Read the model definition and answer for the solid it produces. Units are mm, in the model's axes. A direction names the side the tool comes from. Coordinates: 2 decimals unless noted, no trailing zeros. Loops run counter-clockwise (first coordinate to the right, second up) from the corner with the lowest first, then second, coordinate; pieces in that order, holes last. Notation, with made-up numbers: M -27,69.25 L -16,69.25 A28 ccw -16,97.25 Z; hole C 11.25,15.5 d6. An arc over 180 degrees is marked long. One line per item, written item: value. Start each with the question number.
1. The part is cut by section A-A (x = 113). Write down the section's boundary in (y, z), then the cut area to 3 significant figures.
2. For faces 4 (the face through (120, -11.5, 2)), 5 (the face through (75, 14, 2)), 6 (the face through (-120, -5, 2)), determine the directions among +Z, -Z, +X, -X, +Y, -Y from which every point of the face is accessible in a straight line to the end or side of a thin tool.
3. The part is cut by section B-B (x = -78.5). Write down the section's boundary in (y, z).
4. Consider probe 1 along Y at (x, z) = (113, 2.4); probe 2 along X at (y, z) = (13.5, 2.85); probe 3 along X at (y, z) = (-2, 2). Determine where each line is inside the solid, lowest interval first.
5. Flat-ended cylindrical pins translate along their axes: pin 1 (1.8 mm diameter, centred on x = -127, z = 1.5, fed in from +Y); pin 2 (1 mm diameter, centred on y = 2, z = 2.5, fed in from +X); pin 3 (1.2 mm diameter, centred on x = 92.5, z = 1.5, fed in from -Y); pin 4 (1.5 mm diameter, centred on x = 51, y = 2.5, fed in from +Z). Find the tip coordinate at first contact, or state that the pin passes through.
6. The part is cut by section C-C (z = 3). State how many separate pieces and enclosed holes the cut face has, then the cut area to 3 significant figures.
7. Determine the mould class of faces 1 (the face through (110, -9, 2)), 2 (the face through (-83, -2.5, 2)), 3 (the face through (126, -4, 2)) for opening direction X: +X half, -X half, draft (parallel to the pull), parting line (faces both ways), or undercut.
Autodesk Inventor part; units mm, degrees
ref_plane "YZ Plane" through (0, 0, 0) normal (1, 0, 0) x (0, 1, 0)
ref_plane "XZ Plane" through (0, 0, 0) normal (0, 1, 0) x (-1, 0, 0)
ref_plane "XY Plane" through (0, 0, 0) normal (0, 0, 1) x (1, 0, 0)
sketch "Sketch1" plane through (0, 0, 0) normal (0, 0, 1) x (1, 0, 0)
  line L0 (-130, 16.5) -> (130, 16.5)
  line L1 (130, 16.5) -> (130, -16.5)
  line L2 (130, -16.5) -> (-130, -16.5)
  line L3 (-130, -16.5) -> (-130, 16.5)
  point P0 (0, 0)
  dimension "d0" = 260
  dimension "d1" = 33
  dimension "d2" = 16.5
  dimension "d3" = 130
extrude "Base" add sketch "Sketch1" along normal blind 4
sketch "Sketch2" plane through (0, 0, 4) normal (0, 0, 1) x (1, 0, 0)
  line L0 (130, 16.5) -> (130, -16.5)
  line L1 (-130, 16.5) -> (130, 16.5)
  line L2 (-130, -16.5) -> (-130, 16.5)
  line L3 (130, -16.5) -> (-130, -16.5)
  line L4 (75, 16.5) -> (110, 16.5)
  line L5 (110, 16.5) -> (110, 12.5)
  line L6 (110, 12.5) -> (75, 12.5)
  line L7 (75, 12.5) -> (75, 16.5)
  line L8 (-130, 16.5) -> (55, 16.5)
  line L9 (55, 16.5) -> (55, 12.5)
  line L10 (55, 12.5) -> (-130, 12.5)
  line L11 (-130, 12.5) -> (-130, 16.5)
  line L12 (35, -7.5) -> (55, -7.5)
  line L13 (55, -7.5) -> (55, -16.5)
  line L14 (55, -16.5) -> (35, -16.5)
  line L15 (35, -16.5) -> (35, -7.5)
  line L16 (75, -7.5) -> (110, -7.5)
  line L17 (110, -7.5) -> (110, -16.5)
  line L18 (110, -16.5) -> (75, -16.5)
  line L19 (75, -16.5) -> (75, -7.5)
  line L20 (110, -11.5) -> (130, -11.5)
  line L21 (130, -11.5) -> (130, -16.5)
  line L22 (130, -16.5) -> (110, -16.5)
  line L23 (110, -16.5) -> (110, -11.5)
  line L24 (55, -11.5) -> (75, -11.5)
  line L25 (75, -11.5) -> (75, -16.5)
  line L26 (75, -16.5) -> (55, -16.5)
  line L27 (55, -16.5) -> (55, -11.5)
  point P0 (0, 0)
  dimension "d6" = 35
  dimension "d7" = 4
  dimension "d8" = 0
  dimension "d9" = 20
  dimension "d10" = 185
  dimension "d11" = 4
  dimension "d12" = 0
  dimension "d13" = 0
  dimension "d14" = 20
  dimension "d15" = 20
  dimension "d16" = 9
  dimension "d17" = 0
  dimension "d18" = 165
  dimension "d19" = 35
  dimension "d20" = 9
  dimension "d21" = 0
  dimension "d22" = 20
  dimension "d23" = 20
  dimension "d24" = 5
  dimension "d25" = 20
  dimension "d26" = 5
  dimension "d27" = 0
  dimension "d28" = 0
  dimension "d29" = 0
  dimension "d30" = 0
  dimension "d98" = 20
extrude "StructureMounting" cut sketch "Sketch2" against normal blind 4 contours L0 L3 L17 L20 | L5 L6 L7 L1 | L17 L3 L19 L16 | L9 L10 L2 L1 | L3 L13 L24 L19 | L3 L15 L12 L13
sketch "Sketch4" plane through (0, 0, 4) normal (0, 0, 1) x (1, 0, 0)
  line L0 (55, 12.5) -> (-130, 12.5)
  line L1 (-130, -16.5) -> (-130, 12.5)
  line L2 (35, -16.5) -> (-130, -16.5)
  line L3 (35, -16.5) -> (35, -7.5)
  line L4 (55, 16.5) -> (55, 12.5)
  line L5 (35, -7.5) -> (-130, -16.5)
  line L6 (-130, 3.5) -> (35, 12.5)
  point P0 (0, 0)
  dimension "d42" = 20
  dimension "d43" = 20
extrude "MotorRamp" cut sketch "Sketch4" against normal blind 4
sketch "Sketch5" plane through (0, 0, 4) normal (0, 0, 1) x (1, 0, 0)
  line L0 (110, 12.5) -> (75, 12.5)
  line L1 (75, 12.5) -> (75, 16.5)
  line L2 (94.274, 12.5) -> (98.274, 12.5)
  line L3 (98.274, 12.5) -> (98.274, 2.5)
  line L4 (98.274, 2.5) -> (94.274, 2.5)
  line L5 (94.274, 2.5) -> (94.274, 12.5)
  line L6 (110, 16.5) -> (110, 12.5)
  point P0 (0, 0)
  dimension "d46" = 4
  dimension "d47" = 10
  dimension "d48" = 0
  dimension "d49" = 19.274
  dimension "d100" = 11.726
extrude "LowSleeve" [suppressed]
sketch "Sketch6" plane through (0, 0, 4) normal (0, 0, 1) x (1, 0, 0)
  line L0 (-130, -16.5) -> (-130, 3.5)
  line L1 (-120, -2.5) -> (-105, -2.5)
  line L2 (-105, -2.5) -> (-105, -6.5)
  line L3 (-105, -6.5) -> (-120, -6.5)
  line L4 (-120, -6.5) -> (-120, -2.5)
  line L5 (-90, -2.5) -> (-75, -2.5)
  line L6 (-75, -2.5) -> (-75, -6.5)
  line L7 (-75, -6.5) -> (-90, -6.5)
  line L8 (-90, -6.5) -> (-90, -2.5)
  line L9 (98.274, 2.5) -> (94.274, 2.5)
  line L10 (-106.4171, -4.5) -> (-87.4505, -4.5) construction
  circle A0 centre (-97.5, -4.5) radius 1.25
  point P0 (0, 0)
  dimension "d63" = 15
  dimension "d64" = 4
  dimension "d67" = 30
  dimension "d72" = 10
  dimension "d73" = 10
  dimension "d166" = 2
  dimension "d167" = 2.5
  dimension "d168" = 7.5
extrude "MotorSleeves" cut sketch "Sketch6" against normal blind 4
sketch "Sketch10" plane through (0, 0, 4) normal (0, 0, 1) x (1, 0, 0)
  line L0 (130, 16.5) -> (130, -11.5)
  line L1 (122, 6) -> (130, 6)
  line L2 (130, 6) -> (130, -4)
  line L3 (130, -4) -> (122, -4)
  line L4 (122, -4) -> (122, 6)
  point P0 (0, 0)
  dimension "d109" = 8
  dimension "d110" = 10
  dimension "d111" = 0
  dimension "d112" = 4
extrude "Cabling" cut sketch "Sketch10" against normal blind 4
sketch "Sketch12" plane through (0, 0, 4) normal (0, 0, 1) x (1, 0, 0)
  line L0 (35, 12.5) -> (-130, 3.5)
  line L1 (-0.084, 8.5834) -> (19.8863, 9.6726)
  line L2 (19.8863, 9.6726) -> (20.1041, 5.6786)
  line L3 (20.1041, 5.6786) -> (0.1338, 4.5893)
  line L4 (0.1338, 4.5893) -> (-0.084, 8.5834)
  point P0 (0, 0)
  dimension "d124" = 4
  dimension "d125" = 20
  dimension "d126" = 2
  dimension "d127" = 130
extrude "ESCholder" cut sketch "Sketch12" against normal blind 4
sketch "Sketch13" plane through (0, 0, 4) normal (0, 0, 1) x (1, 0, 0)
  line L0 (55, 16.5) -> (55, 12.5)
  line L1 (55, 12.5) -> (35, 12.5)
  line L2 (35, 12.5) -> (-130, 3.5)
  line L3 (-130, -16.5) -> (35, -7.5)
  line L4 (-30.0123, 6.4502) -> (-26.0182, 6.668)
  line L5 (-26.0182, 6.668) -> (-25.7459, 1.6754)
  line L6 (-25.7459, 1.6754) -> (-29.7399, 1.4576)
  line L7 (-29.7399, 1.4576) -> (-30.0123, 6.4502)
  line L8 (-47.5366, -2.0169) -> (-6.9954, 0.1945) construction
  line L9 (-29.1953, -8.5276) -> (-25.2012, -8.3097)
  line L10 (-25.2012, -8.3097) -> (-25.4736, -3.3171)
  line L11 (-25.4736, -3.3171) -> (-29.4676, -3.535)
  line L12 (-29.4676, -3.535) -> (-29.1953, -8.5276)
  line L13 (20.1041, 5.6786) -> (0.1338, 4.5893)
  line L14 (-27.9377, 5.1382) -> (-27.2725, -7.0585) construction
  circle A0 centre (-27.6051, -0.9601) radius 1.25
  line L15 (49, 10) -> (53, 10)
  line L16 (53, 10) -> (53, 5)
  line L17 (53, 5) -> (49, 5)
  line L18 (49, 5) -> (49, 10)
  line L19 (39.5253, 2.5) -> (63.8345, 2.5) construction
  line L20 (49, -5) -> (53, -5)
  line L21 (53, -5) -> (53, 0)
  line L22 (53, 0) -> (49, 0)
  line L23 (49, 0) -> (49, -5)
  circle A1 centre (51, 2.5) radius 1.25
  point P0 (0, 0)
  dimension "d134" = 2.5
  dimension "d135" = 7.5
  dimension "d136" = 4
  dimension "d137" = 100
  dimension "d140" = 10
  dimension "d151" = 2
  dimension "d152" = 2.5
  dimension "d153" = 4
  dimension "d154" = 5
  dimension "d155" = 2.5
  dimension "d156" = 6
  dimension "d157" = 10
  dimension "d158" = 2.5
  dimension "d159" = 2
extrude "CrossSupports" cut sketch "Sketch13" against normal blind 10
sketch "Sketch14" plane through (0, 0, 4) normal (0, 0, 1) x (1, 0, 0)
  line L0 (110, 12.5) -> (75, 12.5)
  circle A0 centre (113, 8) radius 3
  circle A1 centre (105, 8) radius 3
  point P0 (98.274, 12.5)
  point P1 (0, 0)
  dimension "d141" = 6
  dimension "d142" = 6
  dimension "d143" = 4.5
  dimension "d144" = 4.5
  dimension "d145" = 3
  dimension "d146" = 8
extrude "ESCpowerHoles" cut sketch "Sketch14" against normal blind 10
sketch "Sketch15" plane through (0, 0, 4) normal (0, 0, 1) x (1, 0, 0)
  line L0 (75, -7.5) -> (110, -7.5)
  line L1 (94.274, 2.5) -> (98.274, 2.5)
  line L2 (98.274, 2.5) -> (98.274, -7.5)
  line L3 (98.274, -7.5) -> (94.274, -7.5)
  line L4 (94.274, -7.5) -> (94.274, 2.5)
  point P0 (0, 0)
extrude "HighSleeve" [suppressed]
sketch "Sketch16" plane through (0, 0, 4) normal (0, 0, 1) x (1, 0, 0)
  line L0 (-130, -16.5) -> (-130, 3.5)
  line L1 (-128, 1.5) -> (-126.4, 1.5)
  line L2 (-126.4, 1.5) -> (-126.4, -13.5)
  line L3 (-126.4, -13.5) -> (-128, -13.5)
  line L4 (-128, -13.5) -> (-128, 1.5)
  point P0 (0, 0)
  dimension "d160" = 1.6
  dimension "d161" = 15
  dimension "d162" = 2
  dimension "d163" = 2
extrude "WingLedCutout" cut sketch "Sketch16" against normal blind 10
fillet "ImpactReduction" radius 5 2 edges at (-130, 3.5, 2) (-130, -16.5, 2)
properties part number "ArmOutside"
Answer block:
1. outline: M -11.5,0 L 5,0 L 5,4 L -11.5,4 Z; M 11,0 L 16.5,0 L 16.5,4 L 11,4 Z
1. area: 88.0 mm2
2. face 4: +Z, -Z, +X, -Y
2. face 5: +Z, -Z, +Y
2. face 6: +Z, -Z
3. outline: M -13.69,0 L -6.5,0 L -6.5,4 L -13.69,4 Z; M -2.5,0 L 6.31,0 L 6.31,4 L -2.5,4 Z
4. probe 1: y = -11.5 to 5, 11 to 16.5
4. probe 2: x = 55 to 75, 110 to 130
4. probe 3: x = -130 to -128, -126.4 to -28.3, -26.91 to 49, 53 to 122
5. pin 1: stops at y = 3.64
5. pin 2: stops at x = 122
5. pin 3: stops at y = -7.5
5. pin 4: passes through
6. separate pieces: 1
6. enclosed holes: 13
6. area: 5,050 mm2
7. face 1: undercut
7. face 2: undercut
7. face 3: draft
